```python
from build123d import *

# Parameters (mm, degrees)
F0_R     = 19.223271
F0_R_2   = 31.541662
F1_DEPTH = 33.274


with BuildPart() as f1:
    # F0 (on Top) → F1 (new body)
    with BuildSketch(Plane.XY):
        with BuildLine():
            Line((-8.238693, -14.410725), (-88.9008, -14.410725))
            ThreePointArc((-88.9008, -14.410725), (-94.639506, -25.573134), (-103.286065, -34.670889))
            Line((-103.286065, -34.670889), (4.343193, -34.670889))
            ThreePointArc((4.343193, -34.670889), (-3.225496, -25.334308), (-8.238693, -14.410725))
        make_face()
        with BuildLine():
            ThreePointArc((-103.286065, 34.670889), (-94.639506, 25.573134), (-88.9008, 14.410725))
            Line((-88.9008, 14.410725), (-8.238693, 14.410725))
            ThreePointArc((-8.238693, 14.410725), (-3.225496, 25.334308), (4.343193, 34.670889))
            Line((4.343193, 34.670889), (-103.286065, 34.670889))
        make_face()
        with BuildLine():
            ThreePointArc((4.343193, 34.670889), (-3.225496, 25.334308), (-8.238693, 14.410725))
            ThreePointArc((-8.238693, 14.410725), (-10.451951, 0), (-8.238693, -14.410725))
            ThreePointArc((-8.238693, -14.410725), (-3.225496, -25.334308), (4.343193, -34.670889))
            Line((4.343193, -34.670889), (4.343193, 34.670889))
        make_face()
        with BuildLine():
            ThreePointArc((-88.9008, -14.410725), (-87.092414, -7.305987), (-86.484032, 0))
            ThreePointArc((-86.484032, 0), (-87.092414, 7.305987), (-88.9008, 14.410725))
            ThreePointArc((-88.9008, 14.410725), (-94.639506, 25.573134), (-103.286065, 34.670889))
            Line((-103.286065, 34.670889), (-103.286065, -34.670889))
            ThreePointArc((-103.286065, -34.670889), (-94.639506, -25.573134), (-88.9008, -14.410725))
        make_face()
        with BuildLine():
            Line((-103.286065, -34.670889), (-103.286065, 34.670889))
            ThreePointArc((-103.286065, 34.670889), (-174.829227, 0), (-103.286065, -34.670889))
        make_face()
        with Locations((-130.65663, 0)):
            Circle(F0_R, mode=Mode.SUBTRACT)
        with BuildLine():
            ThreePointArc((85.590833, 0), (56.417298, 44.168002), (4.343193, 34.670889))
            Line((4.343193, 34.670889), (4.343193, -34.670889))
            ThreePointArc((4.343193, -34.670889), (56.417298, -44.168002), (85.590833, 0))
        make_face()
        with Locations((37.569441, 0)):
            Circle(F0_R_2, mode=Mode.SUBTRACT)
    extrude(amount=F1_DEPTH)


solid = f1.part
```
For this review, take the finished solid that the model builds, in its own axes (mm). A direction names the side the tool comes from. Coordinates: 2 decimals unless noted, no trailing zeros. Order: outer loops, then holes, each group sorted by start corner. A loop starts at its lowest first (then second) coordinate and runs counter-clockwise, first axis right, second up. Notation, with made-up numbers: (30, 58) -> (38, 58) arc R23 ccw to (38, 89) -> close; hole circle Ø3 at (24.25, 67.5). An arc over 180 degrees is marked (long way). Use CSV: the item, a comma, the result in double quotes. Start each with the question number.
Item 1: We need section C-C, the plane y = -26.5. Give the boundary of the cut face in (x, z).
Item 2: Wall thickness on probe 1 along Y at (x, z) = (-76.5, 22.5); probe 2 along X at (y, z) = (-10.5, 27); probe 3 along X at (y, z) = (-15, 11): over which ranges is each line inside the solid? List them lowest first.
Item 3: Draft analysis for pull direction X (two halves, no side actions). For faces 5 (the face through (-112.32, 5.77, 16.4)), 6 (the face through (-46, 22, 33.274)), state which applies: pulls with the +X half, pulls with the -X half, needs draft (parallel to the pull), parting line crosses it, or undercut.
Item 4: Insertion check: pin 1 (2 mm diameter, centred on x = 49, z = 20, fed in from -Y); pin 2 (16.5 mm diameter, centred on x = -62.5, z = 17, fed in from -Y); pin 3 (5 mm diameter, centred on x = -120.5, z = 13, fed in from +Y). Each pin has a flat end and moves straight along its axis. Give the tip position at first contact, or say it passes through.
Item 5: For faces 1 (the face through (-49, 14.411, 16)), 2 (the face through (-46, 22, 0)), 3 (the face through (-49, 34.671, 16)), 4 (the face through (-50, -34.671, 16)), list the 3-axis set-ups (+Z, -Z, +X, -X, +Y, -Y) from which the entire face can be reached by the end or side of a thin tool; tool diameter is ignored.
Item 6: We need section A-A, the plane x = -79. Give the boundary of the cut face in (y, z).
Item 7: We need section B-B, the plane z = 21. Give the boundary of the cut face in (x, y).
Derived:
1,outline,"(-166, 0) -> (20.46, 0) -> (20.46, 33.27) -> (-166, 33.27) -> close; (54.68, 0) -> (77.62, 0) -> (77.62, 33.27) -> (54.68, 33.27) -> close"
2,probe 1,"y = -34.67 to -14.41, 14.41 to 34.67"
2,probe 2,"x = -173.56 to -146.76, -114.55 to -87.75, -9.29 to 7.83, 67.31 to 84.43"
2,probe 3,"x = -172.2 to -142.68, -118.63 to 9.82, 65.32 to 83.19"
3,face 5,"undercut"
3,face 6,"needs draft"
4,pin 1,"stops at y = -46.87"
4,pin 2,"stops at y = -34.67"
4,pin 3,"stops at y = 43.5"
5,face 1,"+Z, -Z"
5,face 2,"-Z, +X, -X, +Y, -Y"
5,face 3,"+Z, -Z, +Y"
5,face 4,"+Z, -Z, -Y"
6,outline,"(-34.67, 0) -> (-14.41, 0) -> (-14.41, 33.27) -> (-34.67, 33.27) -> close; (14.41, 0) -> (34.67, 0) -> (34.67, 33.27) -> (14.41, 33.27) -> close"
7,outline,"(-103.29, -34.67) -> (4.34, -34.67) arc R48.02 ccw (long way) to (4.34, 34.67) -> (-103.29, 34.67) arc R44.17 ccw (long way) to start; hole circle Ø38.45 at (-130.66, 0); hole (-88.9, -14.41) -> (-8.24, -14.41) arc R48.02 cw to (-8.24, 14.41) -> (-88.9, 14.41) arc R44.17 cw to (-86.48, 0) arc R44.17 cw to start; hole circle Ø63.08 at (37.57, 0)"
